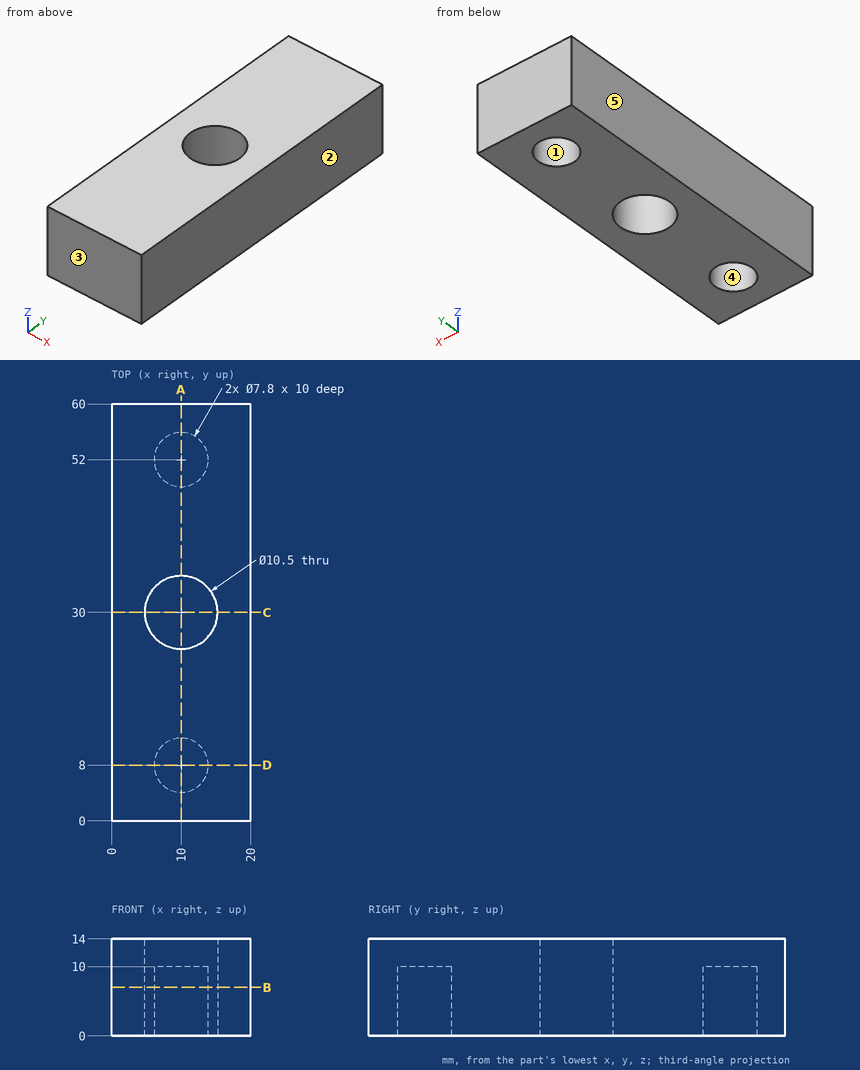
Verification items for this drawing (mm, ordinates from the low corner). A direction names the side the tool comes from. Give positions to 0.01 mm unless a question says otherwise; leave off trailing zeros. Write each loop counter-clockwise with the first axis right and the second up, starting at its lowest first coordinate (ties: lowest second). Pieces come first, ordered by that corner, then holes. Notation, with made-up numbers: (38.25, 72.5) - (56.25, 72.5) arc R10 ccw to (56.25, 76.5) - close; hole circle Ø3 at (87, 28). An arc over 180 degrees is marked (long way). Answer as CSV lines item,"result". Start each with the question number.
1. Set-up check for the marked faces 1 and 2: record each of +Z, -Z, +X, -X, +Y, -Y from which the full face is reachable in a straight line by a thin tool's end or side.
2. Sectioned sample at C-C (y = 30). Record the boundary of the cut face in (x, z), then the cut area to 3 significant figures.
3. Sectioned sample at B-B (z = 7). Record the boundary of the cut face in (x, y).
4. Draft check along Y on the marked faces 3, 4 and 5. Enter one of: pulls with the +Y half, pulls with the -Y half, needs draft (parallel to the pull), parting line crosses it, or undercut.
5. Sectioned sample at D-D (y = 8). Record the boundary of the cut face in (x, z), then the cut area to 3 significant figures.
6. Depth check by flat-ended pin: pin 1 (9.5 mm diameter, centred on x = 10, y = 30, fed in from +Z). Enter the tip coordinate at first touch or a pass-through.
7. Sectioned sample at A-A (x = 10). Record the boundary of the cut face in (y, z).
8. Thickness scan on line 1 (Y direction, x = 10, z = 6.25); line 2 (Y direction, x = 13.25, z = 2.5); line 3 (X direction, y = 26, z = 2.5). Record the ranges inside material, lowest first.
Derived:
1,face 1,"-Z"
1,face 2,"+Z, -Z, +X, +Y, -Y"
2,outline,"(0, 0) - (4.75, 0) - (4.75, 14) - (0, 14) - close; (15.25, 0) - (20, 0) - (20, 14) - (15.25, 14) - close"
2,area,"133 mm²"
3,outline,"(0, 0) - (20, 0) - (20, 60) - (0, 60) - close; hole circle Ø10.5 at (10, 30); hole circle Ø7.8 at (10, 8); hole circle Ø7.8 at (10, 52)"
4,face 3,"pulls with the -Y half"
4,face 4,"undercut"
4,face 5,"needs draft"
5,outline,"(0, 0) - (6.1, 0) - (6.1, 10) - (13.9, 10) - (13.9, 0) - (20, 0) - (20, 14) - (0, 14) - close"
5,area,"202 mm²"
6,pin 1,"through"
7,outline,"(0, 0) - (4.1, 0) - (4.1, 10) - (11.9, 10) - (11.9, 0) - (24.75, 0) - (24.75, 14) - (0, 14) - close; (35.25, 0) - (48.1, 0) - (48.1, 10) - (55.9, 10) - (55.9, 0) - (60, 0) - (60, 14) - (35.25, 14) - close"
8,line 1,"0 to 4.1, 11.9 to 24.75, 35.25 to 48.1, 55.9 to 60"
8,line 2,"0 to 5.84, 10.16 to 25.88, 34.12 to 49.84, 54.16 to 60"
8,line 3,"0 to 6.6, 13.4 to 20"
